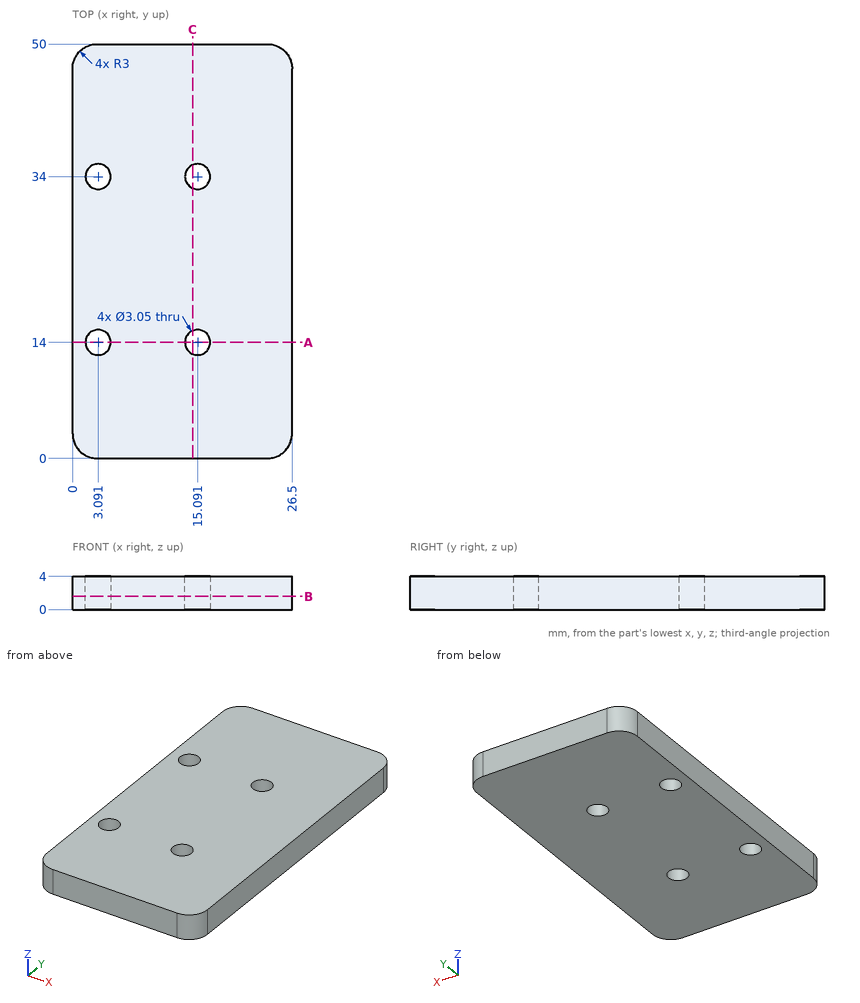
Could you check a few things on this drawing? It's one solid part, dimensions in mm from its lowest x, y, z. Round coordinates to 2 decimals unless told otherwise and drop trailing zeros. Order: outer loops, then holes, each group sorted by start corner. A loop starts at its lowest first (then second) coordinate and runs counter-clockwise, first axis right, second up.
(1) Please list where these lines run through material, in increasing order: line 1 along Y through (x, z) = (15, 1.75); line 2 along Y through (x, z) = (16.25, 3.6); line 3 along X through (y, z) = (33, 2.1).
Response values:
line 1: y = 0 to 12.48, 15.52 to 32.48, 35.52 to 50
line 2: y = 0 to 13.01, 14.99 to 33.01, 34.99 to 50
line 3: x = 0 to 1.94, 4.24 to 13.94, 16.24 to 26.5
(2) I'm going to push a flat-ended pin straight in: pin 1 (2.5 mm diameter, centred on x = 3.09, y = 14, fed in from +Z). Where does the tip first touch, or does it pass through?
Response values:
pin 1: passes through
(3) Imagine slicing it at A-A (y = 14). Write out the boundary of the cut face in (x, z), plus the area to 3 significant figures.
Response values:
outline: (0, 0) - (1.57, 0) - (1.57, 4) - (0, 4) - close; (4.62, 0) - (13.57, 0) - (13.57, 4) - (4.62, 4) - close; (16.62, 0) - (26.5, 0) - (26.5, 4) - (16.62, 4) - close
area: 81.6 mm2
(4) Imagine slicing it at B-B (z = 1.6). Count the separate pieces of the cut face and the enclosed holes in it, plus the area to 3 significant figures.
Response values:
separate pieces: 1
enclosed holes: 4
area: 1,290 mm2
(5) Imagine slicing it at C-C (x = 14.5). Write out the boundary of the cut face in (y, z) (1 decimal).
Response values:
outline: (0, 0) - (12.6, 0) - (12.6, 4) - (0, 4) - close; (15.4, 0) - (32.6, 0) - (32.6, 4) - (15.4, 4) - close; (35.4, 0) - (50, 0) - (50, 4) - (35.4, 4) - close
